Could you check a few things on this model? Use its own coordinates, in mm. A direction names the side the tool comes from. Round coordinates to 2 decimals unless told otherwise and drop trailing zeros. Order: outer loops, then holes, each group sorted by start corner. A loop starts at its lowest first (then second) coordinate and runs counter-clockwise, first axis right, second up. Notation, with made-up numbers: (67, -7) - (116, -7) arc R22 ccw to (116, 14) - close; hole circle Ø9 at (56, 0.5). An arc over 180 degrees is marked (long way). Use one line per item in the form item = value.
Autodesk Fusion 360 part; units mm, degrees
sketch "Horizontal" plane through (0, 0, 0) normal (0, 0, 1) x (1, 0, 0)
  line L0 (40, -20) -> (-40, -20)
  line L1 (-40, 20) -> (40, 20)
  circle A0 centre (40, 0) radius 10
  circle A1 centre (-40, 0) radius 10
  line L2 (20, 0) -> (40, 0) construction
  arc A2 (-40, 20) -> (-40, -20) centre (-40, 0) ccw
  arc A3 (40, -20) -> (40, 20) centre (40, 0) ccw
  dimension "d1" = 80
  dimension "d2" = 40
  dimension "d5" = 40
  dimension "d6" = 40
extrude "Extrude1" add sketch "Horizontal" along normal blind 10
sketch "Vertical" plane through (0, 0, 0) normal (0, 1, 0) x (1, 0, 0)
  line L0 (-20, 0.0761) -> (20, 0.0761)
  line L1 (20, 0.0761) -> (20, -29.9239)
  line L2 (-10, -29.9239) -> (-20, -29.9239)
  line L3 (-20, -29.9239) -> (-20, 0.0761)
  line L4 (-40, 0) -> (-40, -10)
  circle A0 centre (0, -29.9239) radius 10
  arc A1 (-20, -29.9239) -> (20, -29.9239) centre (0, -29.9239) ccw
  dimension "d11" = 40
  dimension "d12" = 30
  dimension "d13" = 20
  dimension "d14" = 20
  dimension "d15" = 20
extrude "Extrude2" add sketch "Vertical" along normal mid plane 40
Item 1: Imagine slicing it at B-B on y = 0. Please give me the cut outline in (x, z), plus the area to 3 significant figures.
Found:
outline = (-60, 0) - (-50, 0) - (-50, 10) - (-60, 10) - close; (-30, 0) - (-20, 0) - (-20, -0.08) - (20, -0.08) - (20, 0) - (30, 0) - (30, 10) - (20, 10) - (20, 29.92) arc R20 ccw to (-20, 29.92) - (-20, 10) - (-30, 10) - close; (50, 0) - (60, 0) - (60, 10) - (50, 10) - close; hole circle Ø20 at (0, 29.92)
area = 1,910 mm2
Item 2: Imagine slicing it at A-A on x = 0. Please give me the cut outline in (y, z).
Found:
outline = (-20, -0.08) - (20, -0.08) - (20, 19.92) - (-20, 19.92) - close; (-20, 39.92) - (20, 39.92) - (20, 49.92) - (-20, 49.92) - close
Item 3: If we mould it in two halves opening along X, with no side actions, what happens to faces 4 (the face through (1, -20, 19)), 5 (the face through (20, 0, 20)), 6 (the face through (-50, 0, 5))? For each: released by +X, released by -X, zero draft, split by the parting line, or undercut.
Found:
face_4 = zero draft
face_5 = released by +X
face_6 = undercut
Item 4: Will these pins go through, and if not, where does the flat tip stop? P1, Ø20, axis at x = 31.5, y = 4, coming from the +Z side; P2, Ø5, axis at y = 13.5, z = 40.5, coming from the -X side; P3, Ø12, axis at x = 47, z = 14.5, coming from the -Y side.
Found:
P1 = 10
P2 = -18.3
P3 = -19.77
Item 5: For faces 1 (the face through (31, 5, 10)), 2 (the face through (-20, 0, 20)), 3 (the face through (0.44, -0.28, 49.92)), which set-ups out of +Z, -Z, +X, -X, +Y, -Y let a thin tool reach every point of the face, with its end or its side?
Found:
face_1 = +Z, +X, +Y, -Y
face_2 = +Z, -X, +Y, -Y
face_3 = +Z, +Y, -Y
Item 6: Imagine slicing it at D-D on z = 27. Please give me the cut outline in (x, y), plus the area to 3 significant figures.
Found:
outline = (-20, -20) - (-9.56, -20) - (-9.56, 20) - (-20, 20) - close; (9.56, -20) - (20, -20) - (20, 20) - (9.56, 20) - close
area = 835 mm2
Item 7: I need wall thicknesses on L1, parallel to Z at x = 0, y = -5; L2, parallel to Y at x = 40, z = 5; L3, parallel to Z at x = 48.5, y = 16. Which ranges of each line are inside material? Lowest first, please.
Found:
L1 = -0.08 to 19.92, 39.92 to 49.92
L2 = -20 to -10, 10 to 20
L3 = 0 to 10
Item 8: Imagine slicing it at C-C on z = 7. Please give me the cut outline in (x, y).
Found:
outline = (-40, -20) - (40, -20) arc R20 ccw to (40, 20) - (-40, 20) arc R20 ccw to start; hole circle Ø20 at (-40, 0); hole circle Ø20 at (40, 0)
